Design review of the part built by this model. Coordinates are the model's own, in mm. A direction names the side the tool comes from. Coordinates: 2 decimals unless noted, no trailing zeros. Loops run counter-clockwise (first coordinate to the right, second up) from the corner with the lowest first, then second, coordinate; pieces in that order, holes last. Notation, with made-up numbers: M 50,-31 L 104,-31 A26 cw 104,7 Z; hole C 66.25,-39 d6. An arc over 180 degrees is marked long. Put each result on its own line as item: value. Start each with the question number.
(1) For faces 4 (the cylindrical face through (46.1, 1.01, -9.14)), 5 (the cylindrical face through (-4.6, 1, 0)), list the 3-axis set-ups (+Z, -Z, +X, -X, +Y, -Y) from which the entire face can be reached by the end or side of a thin tool; tool diameter is ignored.
(2) For probe 1 along Z at (x, y) = (42, 1.6); probe 2 along X at (y, z) = (0.75, -4.75); probe 3 along X at (y, z) = (0.8, 7.25), list the stretches that pass through material, from the lowest coordinate up. Write a range as [from, to].
(3) Take a section at C-C, the plane z = 4.75. Give the boundary of the cut face in (x, y).
(4) Take a section at A-A, the plane z = 0. Give the boundary of the cut face in (x, y).
(5) Take a section at B-B, the plane y = 0.45. Give the boundary of the cut face in (x, z).
(6) The part is to be moulded in two halves that separate along Z. For faces 1 (the flat face through (-10, 1, 0)), 2 (the cylindrical face through (40.85, 0.99, 4.7)), 3 (the cylindrical face through (-9.1, 1.01, -9.14)), say which applies: +Z half, -Z half, draft (parallel to the pull), parting line (faces both ways), or undercut.
```python
from build123d import *

# Parameters (mm, degrees)
SKETCH_1_R          = 1.6
SKETCH_1_R_2        = 1.15
EXTRUDE_1_DEPTH     = 2
FILLET_2_R          = 3
CUT_EXTRUDE_1_DEPTH = 10


with BuildPart() as part:
    # 草图1 → 凸台-拉伸1 (new body)
    with BuildSketch(Plane(origin=(0, 0, 0), x_dir=(1, 0, 0), z_dir=(0, 1, 0))):
        Polygon((-10, 10), (10, 10), (47, 10), (47, -10), (10, -10), (-10, -10), align=None)
        Circle(SKETCH_1_R, mode=Mode.SUBTRACT)
        with Locations((42, -4.75)):
            Circle(SKETCH_1_R_2, mode=Mode.SUBTRACT)
        with Locations((42, 4.75)):
            Circle(SKETCH_1_R_2, mode=Mode.SUBTRACT)
    extrude(amount=EXTRUDE_1_DEPTH)

    # 圆角2
    fillet_2_edges = [part.edges().sort_by_distance(p)[0] for p in [
        (-10, 1, -10),
        (47, 1, -10),
        (47, 1, 10),
        (-10, 1, 10),
    ]]
    fillet(fillet_2_edges, radius=FILLET_2_R)

    # 草图2 → 切除-拉伸1 (cut)
    with BuildSketch(Plane.XZ):
        with BuildLine():
            Line((-3, 1.6), (3, 1.6))
            ThreePointArc((3, 1.6), (4.6, 0), (3, -1.6))
            Line((3, -1.6), (-3, -1.6))
            ThreePointArc((-3, -1.6), (-4.6, 0), (-3, 1.6))
        make_face()
    extrude(amount=-CUT_EXTRUDE_1_DEPTH, mode=Mode.SUBTRACT)


solid = part.part
```
Computed values:
1. face 4: -Z, +X, +Y, -Y
1. face 5: +Y, -Y
2. probe 1: z = [-10, -5.9], [-3.6, 3.6], [5.9, 10]
2. probe 2: x = [-10, 40.85], [43.15, 47]
2. probe 3: x = [-9.99, 46.99]
3. outline: M -10,0 L 40.85,0 L 40.85,2 L -10,2 Z; M 43.15,0 L 47,0 L 47,2 L 43.15,2 Z
4. outline: M -10,0 L -4.6,0 L -4.6,2 L -10,2 Z; M 4.6,0 L 47,0 L 47,2 L 4.6,2 Z
5. outline: M -10,-7 A3 ccw -7,-10 L 44,-10 A3 ccw 47,-7 L 47,7 A3 ccw 44,10 L -7,10 A3 ccw -10,7 Z; hole M -3,-1.6 L 3,-1.6 A1.6 ccw 3,1.6 L -3,1.6 A1.6 ccw Z; hole C 42,-4.75 d2.3; hole C 42,4.75 d2.3
6. face 1: draft
6. face 2: undercut
6. face 3: -Z half
